The listing builds one solid part. Answer for the finished solid, in the listing's coordinates (mm). A direction names the side the tool comes from. Round coordinates to 2 decimals unless told otherwise and drop trailing zeros. Loops run counter-clockwise (first coordinate to the right, second up) from the corner with the lowest first, then second, coordinate; pieces in that order, holes last. Notation, with made-up numbers: (55, 33.25) - (111, 33.25) arc R12 ccw to (111, 46.25) - close; hole circle Ø2 at (65.25, 87.25). An arc over 180 degrees is marked (long way). Write item = value, one per line. Start each with the question number.
1) Section A-A, the plane x = -26 is taken. Determine the outline of the cut face in (y, z).
2) Section D-D, the plane z = 15.75 is taken. Determine the outline of the cut face in (x, y).
3) Section B-B, the plane x = -15 is taken. Determine the outline of the cut face in (y, z), and give its area (3 significant figures).
4) For a pull along X with two mould halves and no side action, classify faces 1 (the flat face through (-19, 18.149, 12)), 2 (the cylindrical face through (-36.15, 17.64, 3.01)), 3 (the cylindrical face through (-24.5, 17.66, 12.57)) as released by +X, released by -X, zero draft, split by the parting line, or undercut.
5) Given pin 1 Ø2 at (y, z) = (9.5, 4.5) entering from -X; pin 2 Ø1.8 at (x, z) = (-26, 12.5) entering from -Y, each flat-ended and moving along its own axis, determine where each tip first touches the part or whether it passes through.
6) Straight lines are drawn through the part: line 1 along Y through (x, z) = (-5, 17.25); line 2 along Z through (x, y) = (-26, 17.7); line 3 along Z through (x, y) = (-26, -36.35). For each, find the intervals that lie inside material, in ascending order.
7) Section C-C, the plane z = 12.5 is taken. Determine the outline of the cut face in (x, y), and give its area (3 significant figures).
8) A tool of negligible diameter and unlimited length cuts with its end or side. For faces 4 (the cylindrical face through (-29.32, -36.36, 15.54)), 5 (the cylindrical face through (0.51, -4.55, 12.57)), 6 (the flat face through (-19, -35.851, 12)), from which of +Z, -Z, +X, -X, +Y, -Y can it reach the whole face along a straight path? Write none if from no direction.
from build123d import *

# Parameters (mm, degrees)
EXTRUIR_L_MINA1_DEPTH = 25
CROQUIS2_R            = 1.5
CORTAR_EXTRUIR1_DEPTH = 1
CROQUIS5_R            = 4.5
CORTAR_EXTRUIR2_DEPTH = 1
CROQUIS6_R            = 1.5
CORTAR_EXTRUIR3_DEPTH = 1
REDONDEO1_R           = 10


with BuildPart() as part:
    # Croquis1 → Extruir-Lámina1 (new body)
    with BuildSketch(Plane.XY):
        Polygon((-39, 17.149283258), (0, 17.149283258), (0, -35.850716742), (-39, -35.850716742), (-39, -36.850716742), (1, -36.850716742), (1, 18.149283258), (-39, 18.149283258), align=None)
    extrude(amount=EXTRUIR_L_MINA1_DEPTH)

    # Croquis2 → Cortar-Extruir1 (cut)
    with BuildSketch(Plane(origin=(0, 18.149283258, 0), x_dir=(1, 0, 0), z_dir=(0, 1, 0))):
        with Locations(Location((-26, -12.5, 0), (0, 0, 180))):
            Circle(CROQUIS2_R)
    extrude(amount=-CORTAR_EXTRUIR1_DEPTH, mode=Mode.SUBTRACT)

    # Croquis5 → Cortar-Extruir2 (cut)
    with BuildSketch(Plane.XZ.offset(36.850716742)):
        with Locations((-26, 12.5)):
            Circle(CROQUIS5_R)
    extrude(amount=-CORTAR_EXTRUIR2_DEPTH, mode=Mode.SUBTRACT)

    # Croquis6 → Cortar-Extruir3 (cut)
    with BuildSketch(Plane(origin=(1, 0, 0), x_dir=(0, 0, -1), z_dir=(1, 0, 0))):
        with Locations(Location((-12.5, -15.650716742, 0), (0, 0, 90))):
            Circle(CROQUIS6_R)
        with Locations(Location((-12.5, -3.050716742, 0), (0, 0, 90))):
            Circle(CROQUIS6_R)
    extrude(amount=-CORTAR_EXTRUIR3_DEPTH, mode=Mode.SUBTRACT)

    # Redondeo1
    redondeo1_edges = [part.edges().sort_by_distance(p)[0] for p in [
        (-39, -36.350716742, 25),
        (-39, 17.649283258, 25),
        (-39, -36.350716742, 0),
        (-39, 17.649283258, 0),
    ]]
    fillet(redondeo1_edges, radius=REDONDEO1_R)


solid = part.part
Geometry check:
q1.outline = (-36.85, 0) - (-35.85, 0) - (-35.85, 8) - (-36.85, 8) - close; (-36.85, 17) - (-35.85, 17) - (-35.85, 25) - (-36.85, 25) - close; (17.15, 0) - (18.15, 0) - (18.15, 11) - (17.15, 11) - close; (17.15, 14) - (18.15, 14) - (18.15, 25) - (17.15, 25) - close
q2.outline = (-38.97, -36.85) - (-29.11, -36.85) - (-29.11, -35.85) - (-38.97, -35.85) - close; (-38.97, 17.15) - (0, 17.15) - (0, -35.85) - (-22.89, -35.85) - (-22.89, -36.85) - (1, -36.85) - (1, 18.15) - (-38.97, 18.15) - close
q3.outline = (-36.85, 0) - (-35.85, 0) - (-35.85, 25) - (-36.85, 25) - close; (17.15, 0) - (18.15, 0) - (18.15, 25) - (17.15, 25) - close
q3.area = 50.0 mm2
q4.face_1 = zero draft
q4.face_2 = released by -X
q4.face_3 = undercut
q5.pin_1 = 0
q5.pin_2 = through
q6.line_1 = -36.85 to -35.85, 17.15 to 18.15
q6.line_2 = 0 to 11, 14 to 25
q6.line_3 = 0 to 8, 17 to 25
q7.outline = (-39, -36.85) - (-30.5, -36.85) - (-30.5, -35.85) - (-39, -35.85) - close; (-39, 17.15) - (-27.5, 17.15) - (-27.5, 18.15) - (-39, 18.15) - close; (-24.5, 17.15) - (0, 17.15) - (0, -1.55) - (1, -1.55) - (1, 18.15) - (-24.5, 18.15) - close; (-21.5, -36.85) - (1, -36.85) - (1, -17.15) - (0, -17.15) - (0, -35.85) - (-21.5, -35.85) - close; (0, -14.15) - (1, -14.15) - (1, -4.55) - (0, -4.55) - close
q7.area = 115 mm2
q8.face_4 = -Y
q8.face_5 = +X, -X
q8.face_6 = +Z, -Z, -X
